from build123d import *

# Parameters (mm, degrees)
SKETCH018_W            = 86
SKETCH018_H            = 115
PAD009_DEPTH           = 60
POCKET008_DEPTH        = 90
LINEARPATTERN005_COUNT = 3
LINEARPATTERN005_PITCH = 17.5
SKETCH020_W            = 84
SKETCH020_H            = 113
POCKET009_DEPTH        = 10
SKETCH021_W            = 84.35487
SKETCH021_H            = 65.313143
POCKET010_DEPTH        = 57


with BuildPart() as part:
    # Sketch018 → Pad009 (new body)
    with BuildSketch(Plane.XY):
        Rectangle(SKETCH018_W, SKETCH018_H)
    extrude(amount=PAD009_DEPTH)

    # Sketch019 (on DatumPlane) → Pocket008 (cut)
    with BuildSketch(Plane(origin=(34, -42.5, 3), x_dir=(1, 0, 0), z_dir=(0, -1, 0))):
        Polygon((-40.082904, 55.425626), (-23.917096, 55.425626), (8.082904, 0), (-8.082904, 0), align=None)
    pocket008 = extrude(amount=-POCKET008_DEPTH, mode=Mode.SUBTRACT)

    # LinearPattern005: Pocket008 ×3
    with Locations(*[(-i * LINEARPATTERN005_PITCH, 0, 0) for i in range(1, LINEARPATTERN005_COUNT)]):
        add(pocket008, mode=Mode.SUBTRACT)

    # Sketch020 (on DatumPlane) → Pocket009 (cut)
    with BuildSketch(Plane.XY.offset(60)):
        Rectangle(SKETCH020_W, SKETCH020_H)
    extrude(amount=-POCKET009_DEPTH, mode=Mode.SUBTRACT)

    # Sketch021 (on DatumPlane) → Pocket010 (cut)
    with BuildSketch(Plane.XY.offset(60)):
        with Locations((-0.938883, 2.685085)):
            Rectangle(SKETCH021_W, SKETCH021_H)
    extrude(amount=-POCKET010_DEPTH, mode=Mode.SUBTRACT)


with BuildPart() as part_1:
    # Body007 placement: moved
    add(part.part.moved(Location((-53, 111, 0))))


solid = part_1.part
Source: CAD feature listing. Evaluate the final solid. Frame: model axes, mm. A direction names the side the tool comes from. Coordinates: 2 decimals unless noted, no trailing zeros. Loops run counter-clockwise (first coordinate to the right, second up) from the corner with the lowest first, then second, coordinate; pieces in that order, holes last. Notation, with made-up numbers: (6.5, 62) - (43.5, 62) arc R12 cw to (43.5, 75) - close; hole circle Ø11 at (82.25, -28). An arc over 180 degrees is marked (long way). One line per item, written item: value. Start each with the question number.
1. Mould query, pull axis Z, two halves, no side actions, for faces 4 (the flat face through (-40.46, 74.68, 26.17)), 5 (the flat face through (-54, 112, 0)), 6 (the flat face through (-19, 81.029, 38)). Classes: pulls with the +Z half, pulls with the -Z half, needs draft (parallel to the pull), parting line crosses it, or undercut.
2. Ray query, L1, parallel to Y at x = -64.5, z = 29.5; L2, parallel to X at y = 75.5, z = 49.5; L3, parallel to Z at x = -32, y = 79.5. Return the intervals inside material, ascending.
3. Section C-C (x = -25.5). Return the cut outline in (y, z), and give its area (3 significant figures).
4. Set-up query: faces 1 (the flat face through (-40.46, 152.34, 26.17)), 2 (the flat face through (-11, 110, 55)), 3 (the flat face through (-83, 146.342, 19)). Return all of +Z, -Z, +X, -X, +Y, -Y with unobstructed straight access to the full face (end or side cutting, diameter ignored); none if empty.
5. Contact query for flat-ended pins moving along their axis: P1, Ø2, axis at x = -62, y = 130, coming from the +Z side; P2, Ø8, axis at y = 131, z = 52.5, coming from the -X side. Output: stop coordinate, or through.
6. Section D-D (y = 127.5). Return the cut outline in (x, z).
7. Section A-A (z = 52.5). Return the cut outline in (x, y), and give its area (3 significant figures).
8. Section B-B (y = 73). Return the cut outline in (x, z).
Verdict:
1. face 4: undercut
1. face 5: pulls with the -Z half
1. face 6: needs draft
2. L1: y = 53.5 to 68.5, 158.5 to 168.5
2. L2: x = -96 to -88.93, -72.76 to -71.43, -55.26 to -53.93, -37.76 to -10
2. L3: z = 0 to 3, 9.21 to 11.52, 39.52 to 50
3. outline: (53.5, 0) - (168.5, 0) - (168.5, 60) - (167.5, 60) - (167.5, 50) - (146.34, 50) - (146.34, 28.26) - (158.5, 28.26) - (158.5, 3) - (68.5, 3) - (68.5, 28.26) - (81.03, 28.26) - (81.03, 50) - (54.5, 50) - (54.5, 60) - (53.5, 60) - close
3. area: 2,080 mm2
4. face 1: none
4. face 2: +Z
4. face 3: +Z, -X
5. P1: stops at z = 3
5. P2: stops at x = -11.76
6. outline: (-96, 0) - (-10, 0) - (-10, 60) - (-11, 60) - (-11, 50) - (-11.76, 50) - (-11.76, 4.46) - (-10.92, 3) - (-96, 3) - close
7. outline: (-96, 53.5) - (-10, 53.5) - (-10, 168.5) - (-96, 168.5) - (-96, 146.34) - (-95, 146.34) - (-95, 167.5) - (-11, 167.5) - (-11, 54.5) - (-95, 54.5) - (-95, 81.03) - (-96, 81.03) - close
7. area: 333 mm2
8. outline: (-96, 0) - (-10, 0) - (-10, 60) - (-11, 60) - (-11, 50) - (-38.05, 50) - (-10.92, 3) - (-27.08, 3) - (-54.22, 50) - (-55.55, 50) - (-28.42, 3) - (-44.58, 3) - (-71.72, 50) - (-73.05, 50) - (-45.92, 3) - (-62.08, 3) - (-89.22, 50) - (-95, 50) - (-95, 60) - (-96, 60) - close
